Can you work these out from the model? Positions are in its coordinate system, mm. Face numbers are marked on the shaded views. A direction names the side the tool comes from. Coordinates: 2 decimals unless noted, no trailing zeros. Order: outer loops, then holes, each group sorted by start corner. A loop starts at its lowest first (then second) coordinate and runs counter-clockwise, first axis right, second up. Notation, with made-up numbers: (14, -26) - (21, -26) arc R20 cw to (21, -22) - close; hole circle Ø11 at (79.5, 31). An arc over 180 degrees is marked (long way). Use a Markdown table: item, result. Add a question column.
(1) For pin 1 Ø8.5 at (x, y) = (-2, 9.5) entering from +Z; pin 2 Ø3 at (x, z) = (-2.5, 12) entering from +Y; pin 3 Ø5 at (x, z) = (2.5, 0.5) entering from +Y, each with a flat end and sliding along its axis, tell me the tip position at first contact or that it passes through.
(2) We'd pull the mould along Z, two halves only. Please class the marked faces 1, 2, 3 and 4: pulls with the +Z half, pulls with the -Z half, needs draft (parallel to the pull), parting line crosses it, or undercut.
(3) If I drill on L1, parallel to X at y = 23.75, z = -4.25; L2, parallel to Z at x = 11, y = 11.5; L3, parallel to Z at x = 3, y = 16.5, over which ranges is the centre line in solid material (lowest first)? Write a range as [from, to].
(4) I want a section at B-B (z = 13.5). List the corners of the cut face in (x, y) for me (1 decimal), and give its area (3 significant figures).
(5) I want a section at A-A (y = 25.25). List the corners of the cut face in (x, z) for me, and give its area (3 significant figures).
(6) I want a section at C-C (z = -7.75). List the corners of the cut face in (x, y) for me.
(7) On a 3-axis mill with a long thin cutter (end or side, diameter ignored), from which of +Z, -Z, +X, -X, +Y, -Y can I reach the whole of each face in a straight line? I mean the marked faces 5, 6 and 7. Say none if no direction works.
(8) I want a section at D-D (y = 2.25). List the corners of the cut face in (x, z) for me, and give its area (3 significant figures).
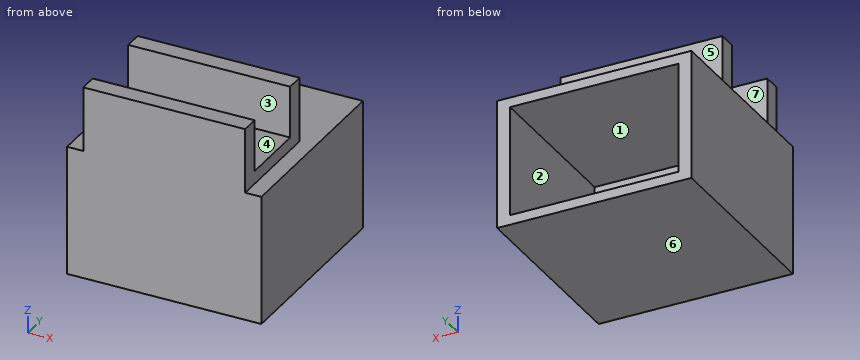
```python
from build123d import *

# Parameters (mm, degrees)
SKETCH_1_W          = 30
SKETCH_1_H          = 20
EXTRUDE_1_DEPTH     = 30
SKETCH_2_W          = 26
SKETCH_2_H          = 17
CUT_EXTRUDE_2_DEPTH = 25
SKETCH_3_W          = 25
SKETCH_3_H          = 16.07
EXTRUDE_2_DEPTH     = 10
SKETCH_4_W          = 8
SKETCH_4_H          = 10.5
CUT_EXTRUDE_3_DEPTH = 45.426074479


with BuildPart() as part:
    # 草图1 → 凸台-拉伸1 (new body)
    with BuildSketch(Plane(origin=(0, 0, 0), x_dir=(1, 0, 0), z_dir=(0, 1, 0))):
        with Locations((-0.371492922, 2.183544304)):
            Rectangle(SKETCH_1_W, SKETCH_1_H)
    extrude(amount=EXTRUDE_1_DEPTH)

    # 草图2 → 切除-拉伸2 (cut)
    with BuildSketch(Plane(origin=(0, 30, 0), x_dir=(1, 0, 0), z_dir=(0, 1, 0))):
        with Locations((-0.371492922, 2.183544304)):
            Rectangle(SKETCH_2_W, SKETCH_2_H)
    extrude(amount=-CUT_EXTRUDE_2_DEPTH, mode=Mode.SUBTRACT)

    # 草图3 → 凸台-拉伸2 (add)
    with BuildSketch(Plane.XY.offset(7.816455696)):
        with Locations((-0.371492922, 8.035)):
            Rectangle(SKETCH_3_W, SKETCH_3_H)
    extrude(amount=EXTRUDE_2_DEPTH)

    # 草图4 → 切除-拉伸3 (cut, through all)
    with BuildSketch(Plane(origin=(12.128507078, 0, 0), x_dir=(0, 0, -1), z_dir=(1, 0, 0))):
        with Locations((-13.816455696, 8.035)):
            Rectangle(SKETCH_4_W, SKETCH_4_H)
    extrude(amount=-CUT_EXTRUDE_3_DEPTH, mode=Mode.SUBTRACT)


solid = part.part
```
Answers follow:
| question | item | result |
|---|---|---|
| 1 | pin 1 | stops at z = 17.82 |
| 1 | pin 2 | stops at y = 16.07 |
| 1 | pin 3 | stops at y = 5 |
| 2 | face 1 | undercut |
| 2 | face 2 | undercut |
| 2 | face 3 | needs draft |
| 2 | face 4 | pulls with the +Z half |
| 3 | L1 | x = [-15.37, -13.37], [12.63, 14.63] |
| 3 | L2 | z = [-12.18, -10.68], [6.32, 9.82] |
| 3 | L3 | z = [-12.18, -10.68], [6.32, 7.82] |
| 4 | outline | (-12.9, 0) - (12.1, 0) - (12.1, 2.8) - (-12.9, 2.8) - close; (-12.9, 13.3) - (12.1, 13.3) - (12.1, 16.1) - (-12.9, 16.1) - close |
| 4 | area | 139 mm² |
| 5 | outline | (-15.37, -12.18) - (14.63, -12.18) - (14.63, 7.82) - (-15.37, 7.82) - close; hole (-13.37, -10.68) - (12.63, -10.68) - (12.63, 6.32) - (-13.37, 6.32) - close |
| 5 | area | 158 mm² |
| 6 | outline | (-15.37, 0) - (14.63, 0) - (14.63, 30) - (12.63, 30) - (12.63, 5) - (-13.37, 5) - (-13.37, 30) - (-15.37, 30) - close |
| 7 | face 5 | +Z, +X, -X, +Y |
| 7 | face 6 | -Z, +X, -X, +Y, -Y |
| 7 | face 7 | +Z, +X, -X |
| 8 | outline | (-15.37, -12.18) - (14.63, -12.18) - (14.63, 7.82) - (12.13, 7.82) - (12.13, 17.82) - (-12.87, 17.82) - (-12.87, 7.82) - (-15.37, 7.82) - close |
| 8 | area | 850 mm² |
